Design review of the part built by this model. Coordinates are the model's own, in mm. Face numbers are marked on the shaded views. A direction names the side the tool comes from. Give positions to 0.01 mm unless a question says otherwise; leave off trailing zeros. Write each loop counter-clockwise with the first axis right and the second up, starting at its lowest first coordinate (ties: lowest second). Pieces come first, ordered by that corner, then holes. Notation, with made-up numbers: (-13, 14) -> (11, 14) arc R33 ccw to (11, 42) -> close; hole circle Ø2 at (-12, 8). An arc over 180 degrees is marked (long way). Use CSV: the item, a comma, the result in double quotes.
```python
from build123d import *

# Parameters (mm, degrees)
DODANIE_WYCI_GNI_CIE1_DEPTH = 1
WYTNIJ_WYCI_GNI_CIE1_REACH  = 13.514
SZKIC8_W                    = 1
SZKIC8_H                    = 6.5
DODANIE_WYCI_GNI_CIE2_DEPTH = 4
WYTNIJ_WYCI_GNI_CIE2_REACH  = 14.148
SZKIC9_W                    = 1
SZKIC9_H                    = 6.5
KONWERTUJ_START             = -3.25
KONWERTUJ_BRY_2_DEPTH       = 6.5
KONWERTUJ_BRY_2_2_DEPTH     = 6.5
WYTNIJ_WYCI_GNI_CIE3_REACH  = 15.041


# Read off the part's stored shape, not the designer's step: Konwertuj bryłę2
with BuildPart() as part:
    # Szkic1 → Dodanie-wyciągnięcie1 (new body)
    with BuildSketch(Plane.XY):
        Polygon((0, -3.25), (0, 3.25), (4.5, 3.25), (4.5, 2.5), (9.5, 2.5), (11, 1.5), (11, -1.5), (9.5, -2.5), (4.5, -2.5), (4.5, -3.25), align=None)
    extrude(amount=DODANIE_WYCI_GNI_CIE1_DEPTH)

    # Szkic2 → Wytnij-wyciągnięcie1 (cut, up to next)
    with BuildSketch(Plane.XY.offset(1), mode=Mode.PRIVATE) as wytnij_wyci_gni_cie1_sk1:
        with BuildLine():
            Line((6.5, 0.979795897), (7.7, 0.734846923))
            ThreePointArc((7.7, 0.734846923), (8.3, 0), (7.7, -0.734846923))
            Line((7.7, -0.734846923), (6.5, -0.979795897))
            ThreePointArc((6.5, -0.979795897), (5.3, 0), (6.5, 0.979795897))
        make_face()
    wytnij_wyci_gni_cie1_tool1 = extrude(wytnij_wyci_gni_cie1_sk1.sketch, amount=-WYTNIJ_WYCI_GNI_CIE1_REACH, mode=Mode.PRIVATE) & part.part
    add(wytnij_wyci_gni_cie1_tool1.solids().sort_by_distance((6.737463, 0, 1))[0], mode=Mode.SUBTRACT)

    # Szkic8 → Dodanie-wyciągnięcie2 (add)
    with BuildSketch(Plane(origin=(0, 0, 0), x_dir=(-1, 0, 0), z_dir=(0, 0, -1))):
        with Locations((-1.5, 0)):
            Rectangle(SZKIC8_W, SZKIC8_H)
    extrude(amount=DODANIE_WYCI_GNI_CIE2_DEPTH)

    # Szkic9 → Wytnij-wyciągnięcie2 (cut, up to next)
    with BuildSketch(Plane(origin=(0, 0, 0), x_dir=(-1, 0, 0), z_dir=(0, 0, -1)), mode=Mode.PRIVATE) as wytnij_wyci_gni_cie2_sk1:
        with Locations((-0.5, 0)):
            Rectangle(SZKIC9_W, SZKIC9_H)
    wytnij_wyci_gni_cie2_tool1 = extrude(wytnij_wyci_gni_cie2_sk1.sketch, amount=-WYTNIJ_WYCI_GNI_CIE2_REACH, mode=Mode.PRIVATE) & part.part
    add(wytnij_wyci_gni_cie2_tool1.solids().sort_by_distance((0.5, 0, 0))[0], mode=Mode.SUBTRACT)

    # Konwertuj bryłę2 outline → Konwertuj bryłę2 (cut)
    with BuildSketch(Plane(origin=(0, 0, 0), x_dir=(1, 0, 0), z_dir=(0, 1, 0)).offset(KONWERTUJ_START)):
        with BuildLine():
            Line((1, -1), (3, -1))
            ThreePointArc((3, -1), (1.585786438, -0.414213562), (1, 1))
            Line((1, 1), (1, -1))
        make_face()
    extrude(amount=KONWERTUJ_BRY_2_DEPTH, mode=Mode.SUBTRACT)

    # Konwertuj bry_2 2 outline → Konwertuj bry_2 2 (add)
    with BuildSketch(Plane(origin=(0, 0, 0), x_dir=(1, 0, 0), z_dir=(0, 1, 0)).offset(KONWERTUJ_START)):
        with BuildLine():
            Line((2, 0), (3, 0))
            ThreePointArc((3, 0), (2.292893219, 0.292893219), (2, 1))
            Line((2, 1), (2, 0))
        make_face()
    extrude(amount=KONWERTUJ_BRY_2_2_DEPTH)

    # Wytnij-wyciągnięcie3: up to this plane
    wytnij_wyci_gni_cie3_end = Plane(origin=(9.5, 2.5, 0), z_dir=(-0.5547001962252293, -0.8320502943378437, 0))
    # Szkic14 → Wytnij-wyciągnięcie3 (cut, up to the surface)
    with BuildSketch(Plane.XZ.offset(2.5), mode=Mode.PRIVATE) as wytnij_wyci_gni_cie3_sk1:
        Polygon((11, 0), (11, 0.5), (9.5, 0), align=None)
    wytnij_wyci_gni_cie3_tool1 = split(extrude(wytnij_wyci_gni_cie3_sk1.sketch, amount=-WYTNIJ_WYCI_GNI_CIE3_REACH, mode=Mode.PRIVATE), bisect_by=wytnij_wyci_gni_cie3_end, keep=Keep.BOTH, mode=Mode.PRIVATE)
    add(wytnij_wyci_gni_cie3_tool1.solids().sort_by_distance((10.5, -2.5, 0.166667))[0], mode=Mode.SUBTRACT)
    # Szkic14 → Wytnij-wyciągnięcie3 (cut, up to the surface)
    with BuildSketch(Plane.XZ.offset(2.5), mode=Mode.PRIVATE) as wytnij_wyci_gni_cie3_sk2:
        Polygon((11, 0.5), (11, 1), (9.5, 1), align=None)
    wytnij_wyci_gni_cie3_tool2 = split(extrude(wytnij_wyci_gni_cie3_sk2.sketch, amount=-WYTNIJ_WYCI_GNI_CIE3_REACH, mode=Mode.PRIVATE), bisect_by=wytnij_wyci_gni_cie3_end, keep=Keep.BOTH, mode=Mode.PRIVATE)
    add(wytnij_wyci_gni_cie3_tool2.solids().sort_by_distance((10.5, -2.5, 0.833333))[0], mode=Mode.SUBTRACT)


solid = part.part
```
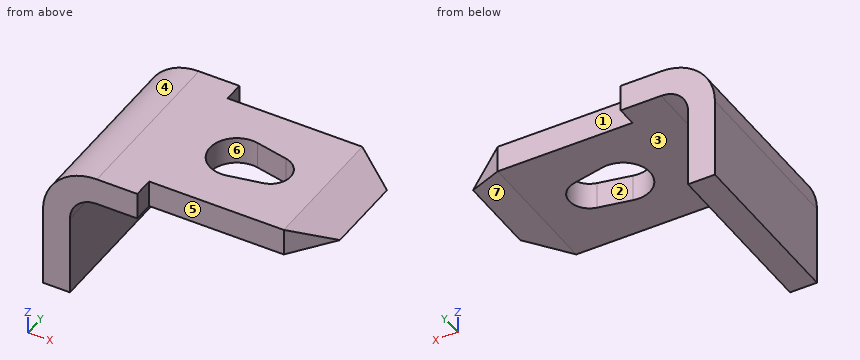
(1) Take a section at A-A (x = 6.3). Write out the cut boundary in (y, z), then the cut area to 3 significant figures.
Established:
outline,"(-2.5, 0) -> (-1, 0) -> (-1, 1) -> (-2.5, 1) -> close; (1, 0) -> (2.5, 0) -> (2.5, 1) -> (1, 1) -> close"
area,"3.00 mm2"
(2) For line 1 along Y through (x, z) = (6.3, 0.4); line 2 along Z through (x, y) = (5, -2); line 3 along X through (y, z) = (1.75, -1.25), list the stretches that pass through material, from the lowest coordinate up. Write a range as [from, to].
Established:
line 1,"y = [-2.5, -1], [1, 2.5]"
line 2,"z = [0, 1]"
line 3,"x = [1, 2]"
(3) Tool access review of the marked faces 1, 2, 3 and 4: name each direction out of +Z, -Z, +X, -X, +Y, -Y from which nothing blocks a thin tool from reaching the whole face with its end or side.
Established:
face 1,"+Z, -Z, +X, +Y"
face 2,"+Z, -Z"
face 3,"-Z, +X, +Y, -Y"
face 4,"+Z, -X, +Y, -Y"
(4) Take a section at D-D (x = 7.5). Write out the cut boundary in (y, z), then the cut area to 3 significant figures.
Established:
outline,"(-2.5, 0) -> (-0.78, 0) -> (-0.78, 1) -> (-2.5, 1) -> close; (0.78, 0) -> (2.5, 0) -> (2.5, 1) -> (0.78, 1) -> close"
area,"3.45 mm2"
(5) Mouldability with a two-part tool opening along X and no side actions: class the marked faces 5, 6 and 7 as +X half, -X half, draft (parallel to the pull), parting line (faces both ways), or undercut.
Established:
face 5,"draft"
face 6,"undercut"
face 7,"+X half"
(6) Clearance check with flat-ended pins moving along their axes: pin 1 (0.6 mm diameter, centred on y = 2.5, z = 0.5, fed in from +X); pin 2 (0.8 mm diameter, centred on x = 7, z = 0.5, fed in from -Y); pin 3 (0.8 mm diameter, centred on y = -3, z = 0.5, fed in from +X). State where each tip first meets the part, or that it passes through.
Established:
pin 1,"stops at x = 9.95"
pin 2,"stops at y = -2.5"
pin 3,"stops at x = 4.5"
(7) Take a section at B-B (y = 0). Write out the cut boundary in (x, z).
Established:
outline,"(1, -4) -> (2, -4) -> (2, -1) arc R1 cw to (3, 0) -> (5.3, 0) -> (5.3, 1) -> (3, 1) arc R2 ccw to (1, -1) -> close; (8.3, 0) -> (9.5, 0) -> (11, 0.5) -> (9.5, 1) -> (8.3, 1) -> close"
(8) Take a section at C-C (y = 2). Write out the cut boundary in (x, z).
Established:
outline,"(1, -4) -> (2, -4) -> (2, -1) arc R1 cw to (3, 0) -> (9.5, 0) -> (10.25, 0.25) -> (10.25, 0.75) -> (9.5, 1) -> (3, 1) arc R2 ccw to (1, -1) -> close"
